Here's how the part is built. I have some questions about the finished solid (model axes, mm). Face numbers are marked on the shaded views. Give positions to 0.01 mm unless a question says otherwise; leave off trailing zeros. Loops run counter-clockwise (first coordinate to the right, second up) from the corner with the lowest first, then second, coordinate; pieces in that order, holes last. Notation, with made-up numbers: (35.5, -21.75) - (88.5, -21.75) arc R20 ccw to (88.5, -10.75) - close; hole circle Ø6 at (-29, 28.5). An arc over 180 degrees is marked (long way). Use a Markdown table: item, result.
from build123d import *

# Parameters (mm, degrees)
SKETCH1_R                 = 6.0325
BOSS_EXTRUDE1_DEPTH       = 12.7
FILLET1_R                 = 0.76
F_8_32_TAPPED_HOLE1_D     = 3.4544
F_8_32_TAPPED_HOLE1_DEPTH = 11.43
F_8_32_TAPPED_HOLE1_TIP   = 1.037806461


with BuildPart() as part:
    # Sketch1 → Boss-Extrude1 (new body)
    with BuildSketch(Plane(origin=(0, 0, 0), x_dir=(1, 0, 0), z_dir=(0, 1, 0))):
        Circle(SKETCH1_R)
    extrude(amount=BOSS_EXTRUDE1_DEPTH)

    # Fillet1
    fillet1_edges = [part.edges().sort_by_distance(p)[0] for p in [
        (-6.0325, 0, 0),
        (-6.0325, 12.7, 0),
    ]]
    fillet(fillet1_edges, radius=FILLET1_R)

    # #8-32 Tapped Hole1
    with Locations(Plane(origin=(0, 12.7, 0), x_dir=(1, 0, 0), z_dir=(0, 1, 0))):
        with Locations((0, 0)):
            Hole(F_8_32_TAPPED_HOLE1_D / 2, depth=F_8_32_TAPPED_HOLE1_DEPTH)
            with Locations((0, 0, -(F_8_32_TAPPED_HOLE1_DEPTH + F_8_32_TAPPED_HOLE1_TIP / 2))):  # 118° drill point
                Cone(0, F_8_32_TAPPED_HOLE1_D / 2, F_8_32_TAPPED_HOLE1_TIP, mode=Mode.SUBTRACT)


solid = part.part
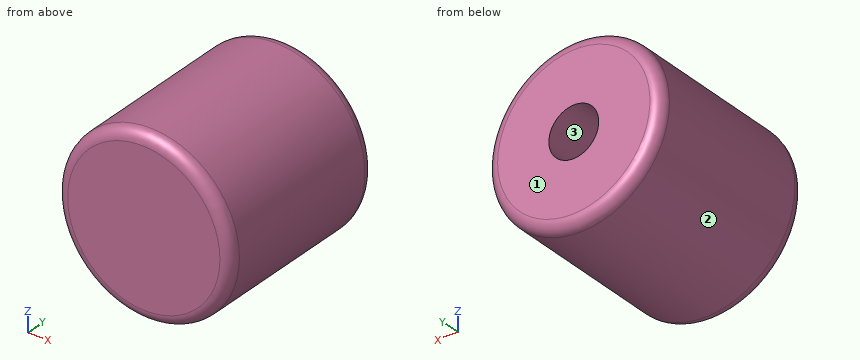
(1) Suppose I cut it at A-A on y = 11.75. Write out the boundary of the cut face in (x, z) (1 decimal), plus the area to 3 significant figures.
A:
| item | result |
|---|---|
| outline | circle Ø12.1 at (0, 0); hole circle Ø3.5 at (0, 0) |
| area | 105 mm2 |
(2) Suppose I cut it at B-B on y = 1. Write out the boundary of the cut face in (x, z) (1 decimal).
A:
| item | result |
|---|---|
| outline | circle Ø12.1 at (0, 0); hole circle Ø2.6 at (0, 0) |
(3) We'd pull the mould along Z, two halves only. Please class the marked faces 1, 2 and 3: pulls with the +Z half, pulls with the -Z half, needs draft (parallel to the pull), parting line crosses it, or undercut.
A:
| item | result |
|---|---|
| face 1 | needs draft |
| face 2 | parting line crosses it |
| face 3 | undercut |
(4) Will these pins go through, and if not, where does the flat tip stop? pin 1 (4 mm diameter, centred on x = -3.5, z = 0, fed in from -Y); pin 2 (1 mm diameter, centred on y = 5.5, z = -3, fed in from +X); pin 3 (1.5 mm diameter, centred on x = -2.5, y = 4.5, fed in from -Z); pin 4 (3 mm diameter, centred on x = 0, z = 0, fed in from +Y).
A:
| item | result |
|---|---|
| pin 1 | y = 0 |
| pin 2 | x = 5.49 |
| pin 3 | z = -5.77 |
| pin 4 | y = 1.13 |
(5) If I drill on line 1 (Z direction, x = 0, y = 6); line 2 (X direction, y = 6, z = -1.5); line 3 (Y direction, x = -3.5, z = 4), over which ranges is the centre line in solid material (lowest first)?
A:
| item | result |
|---|---|
| line 1 | -6.03 to -1.73, 1.73 to 6.03 |
| line 2 | -5.84 to -0.86, 0.86 to 5.84 |
| line 3 | 0 to 12.7 |
